Job drawing, mm, ordinate dimensions from the low corner. One solid piece. Coordinates: 2 decimals unless noted, no trailing zeros. Order: outer loops, then holes, each group sorted by start corner. A loop starts at its lowest first (then second) coordinate and runs counter-clockwise, first axis right, second up. Notation, with made-up numbers: (52, 51.5) - (79, 51.5) arc R28 cw to (79, 81.5) - close; hole circle Ø9 at (30.5, -30). An arc over 180 degrees is marked (long way). Use a Markdown table: item, result. Add a question column.
1) Two-plate mould, pull along Y, no slides. Class the marked faces 1, 2 and 3: +Y half, -Y half, draft (parallel to the pull), parting line (faces both ways), or undercut.
2) Saw through at A-A on y = 19.05. Count the separate pieces of the cut face and the enclosed holes in it, then the cut area to 3 significant figures.
3) Saw through at D-D on z = 48.5. List the corners of the cut face in (x, y), then the cut area to 3 significant figures.
4) Drop flat-ended pins along their axis: P1, Ø1, axis at y = 11, z = 25, coming from the -X side; P2, Ø3, axis at y = 18, z = 17.5, coming from the -X side; P3, Ø1, axis at y = 29.5, z = 24, coming from the +X side; P4, Ø8, axis at y = 32.5, z = 26, coming from the -X side. Give the stop position or say it passes through.
5) Wall check: L1, parallel to X at y = 19, z = 26; L2, parallel to X at y = 13, z = 38 (1 decimal); L3, parallel to Y at x = 38, z = 15. Give the ranges that are in metal, low to high. Write a range as [from, to].
6) Saw through at B-B on z = 30. List the corners of the cut face in (x, y), then the cut area to 3 significant figures.
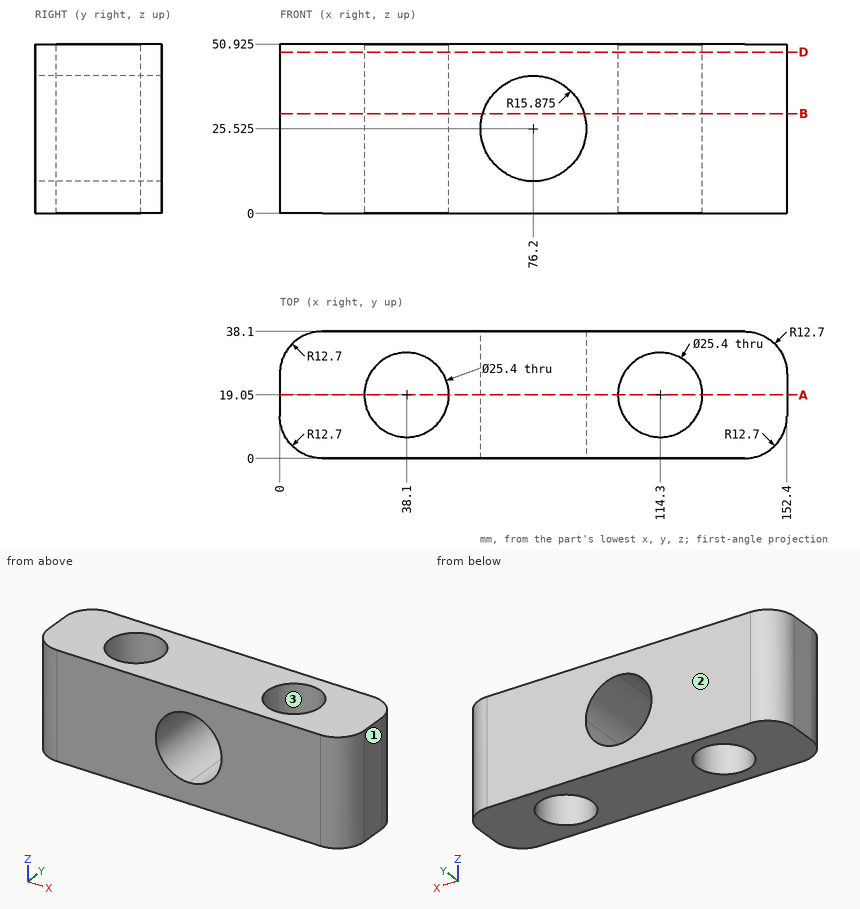
Results are:
| question | item | result |
|---|---|---|
| 1 | face 1 | draft |
| 1 | face 2 | +Y half |
| 1 | face 3 | undercut |
| 2 | separate pieces | 3 |
| 2 | enclosed holes | 1 |
| 2 | area | 4,380 mm2 |
| 3 | outline | (0, 12.7) arc R12.7 ccw to (12.7, 0) - (139.7, 0) arc R12.7 ccw to (152.4, 12.7) - (152.4, 25.4) arc R12.7 ccw to (139.7, 38.1) - (12.7, 38.1) arc R12.7 ccw to (0, 25.4) - close; hole circle Ø25.4 at (38.1, 19.05); hole circle Ø25.4 at (114.3, 19.05) |
| 3 | area | 4,650 mm2 |
| 4 | P1 | x = 0.06 |
| 4 | P2 | x = 0 |
| 4 | P3 | x = 151.88 |
| 4 | P4 | x = 0.38 |
| 5 | L1 | [0, 25.4], [50.8, 60.33], [92.07, 101.6], [127, 152.4] |
| 5 | L2 | [0, 26.9], [49.3, 66.4], [86, 103.1], [125.5, 152.4] |
| 5 | L3 | [0, 6.35], [31.75, 38.1] |
| 6 | outline | (0, 12.7) arc R12.7 ccw to (12.7, 0) - (60.97, 0) - (60.97, 38.1) - (12.7, 38.1) arc R12.7 ccw to (0, 25.4) - close; (91.43, 0) - (139.7, 0) arc R12.7 ccw to (152.4, 12.7) - (152.4, 25.4) arc R12.7 ccw to (139.7, 38.1) - (91.43, 38.1) - close; hole circle Ø25.4 at (38.1, 19.05); hole circle Ø25.4 at (114.3, 19.05) |
| 6 | area | 3,490 mm2 |
